Input: dimensioned drawing with shaded views. Units: mm. Origin: part minimum x, y, z. A direction names the side the tool comes from. Give positions to 0.01 mm unless a question says otherwise; leave off trailing zeros. Write each loop counter-clockwise with the first axis right and the second up, starting at its lowest first coordinate (ties: lowest second). Pieces come first, ordered by that corner, then holes. Notation, with made-up numbers: (63.5, 19.5) - (107.5, 19.5) arc R10 cw to (107.5, 36.5) - close; hole circle Ø4 at (26.5, 16.25). An arc over 180 degrees is marked (long way). Answer as CSV lines item,"result".
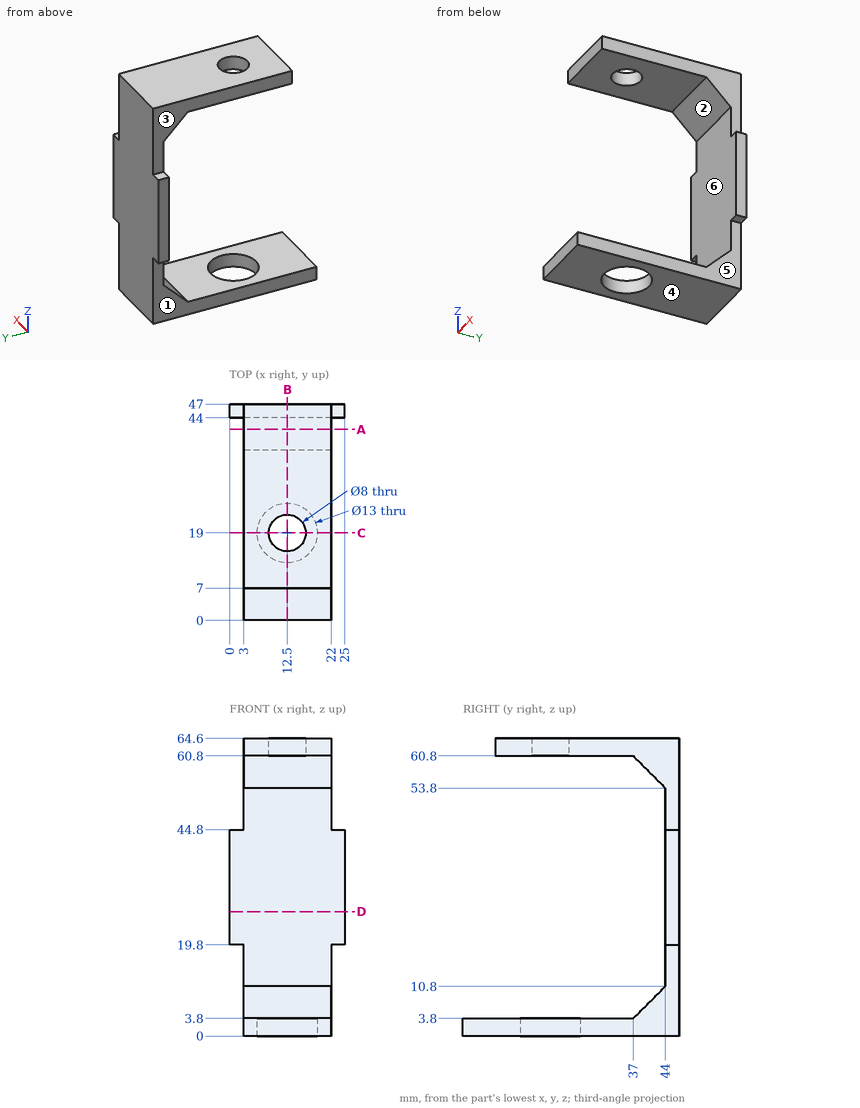
Item 1: Ray query, line 1 (Y direction, x = 12.5, z = 1.9); line 2 (Y direction, x = 12.5, z = 63.5); line 3 (Z direction, x = 19, y = 22.5). Return the intervals inside material, ascending. Write a range as from..to.
The answers:
line 1,"0..12.5, 25.5..47"
line 2,"7..15, 23..47"
line 3,"0..3.8, 60.8..64.6"
Item 2: Cut plane A-A on y = 41.5. Return the cut outline in (x, z), plus the area to 3 significant figures.
The answers:
outline,"(3, 0) - (22, 0) - (22, 8.3) - (3, 8.3) - close; (3, 56.3) - (22, 56.3) - (22, 64.6) - (3, 64.6) - close"
area,"315 mm²"
Item 3: Contact query for flat-ended pins moving along their axis: pin 1 (6 mm diameter, centred on y = 23, z = 57.5, fed in from -X) (3 decimals); pin 2 (2.5 mm diameter, centred on x = 23.5, y = 45, fed in from +Z); pin 3 (10.5 mm diameter, centred on x = 12.5, y = 19, fed in from -Z); pin 4 (1 mm diameter, centred on x = 13.5, z = 34.5, fed in from -Y). Output: stop coordinate, or through.
The answers:
pin 1,"through"
pin 2,"z = 44.8"
pin 3,"z = 60.8"
pin 4,"y = 44"
Item 4: Reachability of the marked faces 1, 2 and 3 from +Z, -Z, +X, -X, +Y, -Y: full face, straight path, thin tool, end or side. Return the list, or none.
The answers:
face 1,"-Z, -X, +Y, -Y"
face 2,"+X, -X, -Y"
face 3,"+Z, -X, +Y, -Y"
Item 5: Cut plane B-B on x = 12.5. Return the cut outline in (y, z).
The answers:
outline,"(0, 0) - (12.5, 0) - (12.5, 3.8) - (0, 3.8) - close; (7, 60.8) - (15, 60.8) - (15, 64.6) - (7, 64.6) - close; (23, 60.8) - (37, 60.8) - (44, 53.8) - (44, 10.8) - (37, 3.8) - (25.5, 3.8) - (25.5, 0) - (47, 0) - (47, 64.6) - (23, 64.6) - close"
Item 6: Mould query, pull axis Z, two halves, no side actions, for the marked faces 4, 5 and 6. Classes: +Z half, -Z half, draft (parallel to the pull), parting line (faces both ways), or undercut.
The answers:
face 4,"-Z half"
face 5,"draft"
face 6,"undercut"
Item 7: Cut plane C-C on y = 19. Return the cut outline in (x, z), plus the area to 3 significant figures.
The answers:
outline,"(3, 0) - (6, 0) - (6, 3.8) - (3, 3.8) - close; (3, 60.8) - (8.5, 60.8) - (8.5, 64.6) - (3, 64.6) - close; (16.5, 60.8) - (22, 60.8) - (22, 64.6) - (16.5, 64.6) - close; (19, 0) - (22, 0) - (22, 3.8) - (19, 3.8) - close"
area,"64.6 mm²"
Item 8: Cut plane D-D on z = 27. Return the cut outline in (x, y), plus the area to 3 significant figures.
The answers:
outline,"(0, 44) - (25, 44) - (25, 47) - (0, 47) - close"
area,"75.0 mm²"
